from build123d import *

# Parameters (mm, degrees)
SKETCH2_W           = 19
SKETCH2_H           = 19
SKETCH2_W_2         = 15
SKETCH2_H_2         = 15
SKETCH3_W           = 180
SKETCH3_H           = 150
BOSS_EXTRUDE1_DEPTH = 10
BOSS_EXTRUDE1_TAPER = 40
SKETCH4_W           = 14.282717188
SKETCH4_H           = 133.218007376
BOSS_EXTRUDE2_DEPTH = 180
BOSS_EXTRUDE2_TAPER = 2


with BuildPart() as part:
    # Sweep-Thin1: sweep along a curve in space
    with BuildLine() as sweep_thin1_path:
        Line((0, 0, 0), (-70, 0, 0))
        ThreePointArc((-70, 0, 0), (-77.071067812, -2.928932188, 0), (-80, -10, 0))
        Line((-80, -10, 0), (-80, -90, 0))
        ThreePointArc((-80, -90, 0), (-77.071067812, -97.071067812, 0), (-70, -100, 0))
        Line((-70, -100, 0), (50, -100, 0))
        ThreePointArc((50, -100, 0), (57.071067812, -100, 2.928932188), (60, -100, 10))
        Line((60, -100, 10), (60, -100, 190))
        ThreePointArc((60, -100, 190), (57.071067812, -100, 197.071067812), (50, -100, 200))
        Line((50, -100, 200), (-70, -100, 200))
        ThreePointArc((-70, -100, 200), (-77.071067812, -97.071067812, 200), (-80, -90, 200))
        Line((-80, -90, 200), (-80, -10, 200))
        ThreePointArc((-80, -10, 200), (-77.071067812, -2.928932188, 200), (-70, 0, 200))
        Line((-70, 0, 200), (60, 0, 200))
    # Sketch2 → Sweep-Thin1 (sweep)
    with BuildSketch(Plane(origin=(0, 0, 0), x_dir=(0, 0, -1), z_dir=(1, 0, 0))):
        Rectangle(SKETCH2_W, SKETCH2_H)
        Rectangle(SKETCH2_W_2, SKETCH2_H_2, mode=Mode.SUBTRACT)
    sweep(path=sweep_thin1_path.line)

    # Sketch3 → Boss-Extrude1 (add)
    with BuildSketch(Plane.XY.offset(209.5)):
        with Locations((-15.849049542, -51.188068464)):
            Rectangle(SKETCH3_W, SKETCH3_H)
    extrude(amount=BOSS_EXTRUDE1_DEPTH, taper=BOSS_EXTRUDE1_TAPER)

    # Sketch4 → Boss-Extrude2 (add)
    with BuildSketch(Plane.XY.offset(219.5)):
        with Locations((58.618595553, -51.188068464)):
            Rectangle(SKETCH4_W, SKETCH4_H)
    extrude(amount=BOSS_EXTRUDE2_DEPTH, taper=BOSS_EXTRUDE2_TAPER)


solid = part.part
Geometry check sheet. Reference: the model listing, model coordinates, mm. A direction names the side the tool comes from. Round coordinates to 2 decimals unless told otherwise and drop trailing zeros. Order: outer loops, then holes, each group sorted by start corner. A loop starts at its lowest first (then second) coordinate and runs counter-clockwise, first axis right, second up. Notation, with made-up numbers: M 8,-32.75 L 27,-32.75 A34 cw 27,1.25 Z; hole C 54,56.25 d9. An arc over 180 degrees is marked long. Write each question's results on one line, items separated by ' | '. Start each with the question number.
1. Material ranges on L1, parallel to Z at x = -80.5, y = -80.5; L2, parallel to Y at x = 27.5, z = 202; L3, parallel to Z at x = -15, y = -36.5, recorded low to high. Write a range as from..to.
2. Draft check along Y on faces 1 (the face through (-17.1, 19.7, 214.4)), 2 (the face through (60, 0, 192)), 3 (the face through (52.5, -100, 101)). Enter one of: pulls with the +Y half, pulls with the -Y half, needs draft (parallel to the pull), parting line crosses it, or undercut.
3. Cross-section at A-A on y = -58. Record the boundary of the cut face in (x, z), plus the area to 3 significant figures.
4. Cross-section at B-B on x = 22. Record the boundary of the cut face in (y, z).
5. Cross-section at C-C on z = 151.5. Record the boundary of the cut face in (x, y), plus the area to 3 significant figures.
6. Set-up check for faces 4 (the face through (-35, 9.5, 0)), 5 (the face through (-89.5, -49, 200)), 6 (the face through (-35, -7.5, 0)), 7 (the face through (-83.636, 3.939, 0.133)), 8 (the face through (-87.5, -51, 0)): record each of +Z, -Z, +X, -X, +Y, -Y from which the full face is reachable in a straight line by a thin tool's end or side.
7. Cross-section at D-D on x = -48. Give the number of separate pieces and of enclosed holes in the cut face, plus the area to 3 significant figures.
8. Go/stop test with flat-tipped pins: P1, Ø5.5, axis at y = -100, z = 60.5, coming from the +X side; P2, Ø5, axis at y = -17.5, z = 307.5, coming from the -X side; P3, Ø12, axis at y = -52, z = -2, coming from the -X side. Record where each tip stops, or that it passes through.
Resolved:
1) L1: -9.5..-7.5, 7.5..9.5, 190.5..192.5, 207.5..219.5 | L2: -109.5..-107.5, -92.5..-90.5, -9.5..-7.5, 7.5..9.5 | L3: 209.5..219.5
2) face 1: pulls with the +Y half | face 2: needs draft | face 3: undercut
3) outline: M -105.85,209.5 L -89.5,209.5 L -89.5,190.5 L -70.5,190.5 L -70.5,209.5 L 74.15,209.5 L 65.76,219.5 L 59.47,399.5 L 57.76,399.5 L 51.48,219.5 L -97.46,219.5 Z; M -89.5,-9.5 L -70.5,-9.5 L -70.5,9.5 L -89.5,9.5 Z; hole M -87.5,-7.5 L -72.5,-7.5 L -72.5,7.5 L -87.5,7.5 Z; hole M -87.5,192.5 L -72.5,192.5 L -72.5,207.5 L -87.5,207.5 Z | area: 3,430 mm2
4) outline: M -126.19,209.5 L -109.5,209.5 L -109.5,190.5 L -90.5,190.5 L -90.5,209.5 L -9.5,209.5 L -9.5,190.5 L 9.5,190.5 L 9.5,209.5 L 23.81,209.5 L 15.42,219.5 L -117.8,219.5 Z; M -109.5,-9.5 L -90.5,-9.5 L -90.5,9.5 L -109.5,9.5 Z; hole M -107.5,-7.5 L -92.5,-7.5 L -92.5,7.5 L -107.5,7.5 Z; hole M -107.5,192.5 L -92.5,192.5 L -92.5,207.5 L -107.5,207.5 Z; hole M -7.5,192.5 L 7.5,192.5 L 7.5,207.5 L -7.5,207.5 Z
5) outline: M 50.5,-109.5 L 69.5,-109.5 L 69.5,-90.5 L 50.5,-90.5 Z; hole M 52.5,-107.5 L 67.5,-107.5 L 67.5,-92.5 L 52.5,-92.5 Z | area: 136 mm2
6) face 4: -Z, +X, -X, +Y | face 5: -Z, -X, +Y, -Y | face 6: +X | face 7: -Z, -X, +Y | face 8: none
7) separate pieces: 3 | enclosed holes: 4 | area: 1,960 mm2
8) P1: x = 69.5 | P2: x = 54.46 | P3: x = -89.5
